Work out the finished part from the listing and answer in its coordinate system (mm). Coordinates: 2 decimals unless noted, no trailing zeros. Order: outer loops, then holes, each group sorted by start corner. A loop starts at its lowest first (then second) coordinate and runs counter-clockwise, first axis right, second up. Notation, with made-up numbers: (79.5, 11.25) - (136.5, 11.25) arc R23 cw to (136.5, 24.25) - close; hole circle Ø10 at (25, 55). An arc over 180 degrees is marked (long way). Answer as a JSON object with one key per item and string values. Group by question number.
1) Section D-D (x = 7) is taken. Give the vertices of the cut face in (y, z), plus the area to 3 significant figures.
2) Each of these flat-tipped pins is pushed along its axis until it touches: P1, Ø3, axis at x = -7.5, z = 19, coming from the -Y side; P2, Ø5, axis at x = 2.5, y = 2.5, coming from the +Z side; P3, Ø1.5, axis at y = 2, z = 13, coming from the -X side. Where does it stop, or does it pass through?
3) Section B-B (x = 16) is taken. Give the vertices of the cut face in (y, z).
4) Find the intervals of material crossed by line 1 along Y through (x, z) = (-13, 8.75); line 2 along Z through (x, y) = (-17, -2); line 3 along Z through (x, y) = (24, -4), in increasing order.
5) Section A-A (y = 3.75) is taken. Count the separate pieces of the cut face and the enclosed holes in it, plus the area to 3 significant figures.
from build123d import *

# Parameters (mm, degrees)
F1_DEPTH = 6.35
F2_DEPTH = 1.143
F0_R     = 0.5376774343
F3_DEPTH = 2.54


# Not quite as in the source:
# - a feature names something its author has since deleted; it is built from what else it names


with BuildPart() as f1:
    # F0 (on Front) → F1 (new body, symmetric)
    with BuildSketch(Plane.XZ):
        with BuildLine():
            Line((-23.957899441, 10.4580381471), (-18.3417778462, 24.3978608632))
            ThreePointArc((-18.3417778462, 24.3978608632), (-24.508682548, 21.9832418882), (-30.3090570475, 18.7868761299))
            ThreePointArc((-30.3090570475, 18.7868761299), (-30.4688345425, 18.7669734191), (-30.6283324456, 18.7449419699))
            ThreePointArc((-30.6283324456, 18.7449419699), (-33.5331514259, 15.8401229896), (-30.6283324456, 12.9353040093))
            ThreePointArc((-30.6283324456, 12.9353040093), (-29.7623700905, 12.8471763438), (-28.8964077355, 12.9353040093))
            ThreePointArc((-28.8964077355, 12.9353040093), (-26.4593844973, 11.6324177359), (-23.957899441, 10.4580381471))
        make_face()
    extrude(amount=F1_DEPTH, both=True)



with BuildPart() as f1b:
    # F0 (on Front) → F1, piece 2 (new body, symmetric)
    with BuildSketch(Plane.XZ):
        with BuildLine():
            Line((-18.3417778462, 8.3667041198), (-12.1646409942, 25.9439263056))
            ThreePointArc((-12.1646409942, 25.9439263056), (-14.2076271577, 25.5232665303), (-16.2316225469, 25.0190941641))
            Line((-16.2316225469, 25.0190941641), (-22.1410569955, 9.7018790977))
            Line((-22.1410569955, 9.7018790977), (-18.3417778462, 8.3667041198))
        make_face()
    extrude(amount=F1_DEPTH, both=True)


with BuildPart() as f1c:
    # F0 (on Front) → F1, piece 3 (new body, symmetric)
    with BuildSketch(Plane.XZ):
        with BuildLine():
            Line((1.8068482134, 6.1805279437), (6.278092768, 25.9439263056))
            ThreePointArc((6.278092768, 25.9439263056), (4.5833562732, 26.2272072808), (2.8800089407, 26.4530119809))
            Line((2.8800089407, 26.4530119809), (-1.8782013648, 5.999318733))
            Line((-1.8782013648, 5.999318733), (1.8068482134, 6.1805279437))
        make_face()
        with BuildLine():
            Line((-1.8782013648, 5.999318733), (2.8800089407, 26.4530119809))
            Line((2.8800089407, 26.4530119809), (0.4476490102, 26.6745825214))
            Line((0.4476490102, 26.6745825214), (-5.0909425313, 6.0502526163))
            ThreePointArc((-5.0909425313, 6.0502526163), (-3.4849571687, 6.0004872294), (-1.8782013648, 5.999318733))
        make_face()
    extrude(amount=F1_DEPTH, both=True)


with BuildPart() as f1d:
    # F0 (on Front) → F1, piece 4 (new body, symmetric)
    with BuildSketch(Plane.XZ):
        with BuildLine():
            Line((8.4127366642, 7.1570997269), (11.4288211982, 24.7124430234))
            ThreePointArc((11.4288211982, 24.7124430234), (9.992896211, 25.1131857412), (8.5458304529, 25.4716212117))
            Line((8.5458304529, 25.4716212117), (5.5570962218, 6.6305751818))
            Line((5.5570962218, 6.6305751818), (8.4127366642, 7.1570997269))
        make_face()
    extrude(amount=F1_DEPTH, both=True)


with BuildPart() as f1e:
    # F0 (on Front) → F1, piece 5 (new body, symmetric)
    with BuildSketch(Plane.XZ):
        with BuildLine():
            Line((15.3388230563, 9.1300772804), (17.0374851182, 22.6934409017))
            ThreePointArc((17.0374851182, 22.6934409017), (15.6698818595, 23.2551052755), (14.2865132328, 23.7767342476))
            Line((14.2865132328, 23.7767342476), (12.4090739429, 8.1711044117))
            Line((12.4090739429, 8.1711044117), (15.3388230563, 9.1300772804))
        make_face()
    extrude(amount=F1_DEPTH, both=True)


with BuildPart() as f1f:
    # F0 (on Front) → F1, piece 6 (new body, symmetric)
    with BuildSketch(Plane.XZ):
        with BuildLine():
            Line((21.0198694331, 18.0883333087), (21.0198694322, 20.7808247964))
            ThreePointArc((21.0198694322, 20.7808247964), (20.069859076, 21.2762433466), (19.1096116707, 21.7515160445))
            Line((19.1096116707, 21.7515160445), (17.6402366731, 10.0189484933))
            ThreePointArc((17.6402366731, 10.0189484933), (19.3434832269, 10.757776133), (21.0198694351, 11.5556761172))
            Line((21.0198694351, 11.5556761172), (21.0198694343, 14.3284648657))
            Line((21.0198694343, 14.3284648657), (21.0198694331, 18.0883333087))
        make_face()
        Polygon((21.0198694343, 14.3284648657), (28.0039037731, 15.6337103452), (21.0198694331, 18.0883333087), align=None)
    extrude(amount=F1_DEPTH, both=True)


with BuildPart() as f1_1:
    add(f1.part)

    add(f1b.part)  # F2 merges F1b

    add(f1c.part)  # F2 merges F1c

    add(f1d.part)  # F2 merges F1d

    add(f1e.part)  # F2 merges F1e

    add(f1f.part)  # F2 merges F1f
    # F0 (on Front) → F2 (join, symmetric)
    with BuildSketch(Plane.XZ):
        with BuildLine():
            Line((-12.1127719974, 6.8447730539), (-5.6567463208, 26.7153601349))
            ThreePointArc((-5.6567463208, 26.7153601349), (-6.3478066879, 26.6736702184), (-7.0382347309, 26.6225664263))
            Line((-7.0382347309, 26.6225664263), (-8.9119801903, 26.3745176413))
            Line((-8.9119801903, 26.3745176413), (-16.2316225469, 7.7613705689))
            ThreePointArc((-16.2316225469, 7.7613705689), (-14.1813025903, 7.2621558762), (-12.1127719974, 6.8447730539))
        make_face()
        with BuildLine():
            Line((-5.0909425313, 6.0502526163), (0.4476490102, 26.6745825214))
            ThreePointArc((0.4476490102, 26.6745825214), (-1.1501754418, 26.7562261377), (-2.7497784488, 26.787513187))
            Line((-2.7497784488, 26.787513187), (-9.4000246121, 6.4253498282))
            ThreePointArc((-9.4000246121, 6.4253498282), (-9.0947770245, 6.3870993561), (-8.7893130258, 6.3506173901))
            ThreePointArc((-8.7893130258, 6.3506173901), (-7.91449717, 6.2560428931), (-7.0382347309, 6.1759725811))
            ThreePointArc((-7.0382347309, 6.1759725811), (-6.0651659933, 6.1041697642), (-5.0909425313, 6.0502526163))
        make_face()
        with BuildLine():
            Line((-9.4000246121, 6.4253498282), (-2.7497784488, 26.787513187))
            ThreePointArc((-2.7497784488, 26.787513187), (-2.8593531847, 26.7878123797), (-2.968928311, 26.7878752202))
            Line((-2.968928311, 26.7878752202), (-5.6567463208, 26.7153601349))
            Line((-5.6567463208, 26.7153601349), (-12.1127719974, 6.8447730539))
            ThreePointArc((-12.1127719974, 6.8447730539), (-10.7591081046, 6.6175349855), (-9.4000246121, 6.4253498282))
        make_face()
        with BuildLine():
            ThreePointArc((-18.3417778462, 8.3667041198), (-17.2898277228, 8.0531349816), (-16.2316225469, 7.7613705689))
            Line((-16.2316225469, 7.7613705689), (-8.9119801903, 26.3745176413))
            Line((-8.9119801903, 26.3745176413), (-12.1646409942, 25.9439263056))
            Line((-12.1646409942, 25.9439263056), (-18.3417778462, 8.3667041198))
        make_face()
        with BuildLine():
            Line((5.5570962218, 6.6305751818), (8.5458304529, 25.4716212117))
            Line((8.5458304529, 25.4716212117), (6.278092768, 25.9439263056))
            Line((6.278092768, 25.9439263056), (1.8068482134, 6.1805279437))
            ThreePointArc((1.8068482134, 6.1805279437), (3.6859738146, 6.3722062161), (5.5570962218, 6.6305751818))
        make_face()
        with BuildLine():
            Line((12.4090739429, 8.1711044117), (14.2865132328, 23.7767342476))
            Line((14.2865132328, 23.7767342476), (11.4288211982, 24.7124430234))
            Line((11.4288211982, 24.7124430234), (8.4127366642, 7.1570997269))
            ThreePointArc((8.4127366642, 7.1570997269), (10.4207473928, 7.62531299), (12.4090739429, 8.1711044117))
        make_face()
        with BuildLine():
            Line((17.6402366731, 10.0189484933), (19.1096116707, 21.7515160445))
            Line((19.1096116707, 21.7515160445), (17.0374851182, 22.6934409017))
            Line((17.0374851182, 22.6934409017), (15.3388230563, 9.1300772804))
            ThreePointArc((15.3388230563, 9.1300772804), (16.4946911486, 9.5611495909), (17.6402366731, 10.0189484933))
        make_face()
        with BuildLine():
            Line((-22.1410569955, 9.7018790977), (-16.2316225469, 25.0190941641))
            ThreePointArc((-16.2316225469, 25.0190941641), (-17.2900631098, 24.7199003867), (-18.3417778462, 24.3978608632))
            Line((-18.3417778462, 24.3978608632), (-23.957899441, 10.4580381471))
            ThreePointArc((-23.957899441, 10.4580381471), (-23.0529803303, 10.0715440095), (-22.1410569955, 9.7018790977))
        make_face()
    extrude(amount=F2_DEPTH, both=True)

    # F0 (on Front) → F3 (join, symmetric)
    with BuildSketch(Plane.XZ):
        with BuildLine():
            Line((-22.1410569955, 9.7018790977), (-16.2316225469, 25.0190941641))
            ThreePointArc((-16.2316225469, 25.0190941641), (-17.2900631098, 24.7199003867), (-18.3417778462, 24.3978608632))
            Line((-18.3417778462, 24.3978608632), (-23.957899441, 10.4580381471))
            ThreePointArc((-23.957899441, 10.4580381471), (-23.0529803303, 10.0715440095), (-22.1410569955, 9.7018790977))
        make_face()
        with BuildLine():
            ThreePointArc((-18.3417778462, 8.3667041198), (-17.2898277228, 8.0531349816), (-16.2316225469, 7.7613705689))
            Line((-16.2316225469, 7.7613705689), (-8.9119801903, 26.3745176413))
            Line((-8.9119801903, 26.3745176413), (-12.1646409942, 25.9439263056))
            Line((-12.1646409942, 25.9439263056), (-18.3417778462, 8.3667041198))
        make_face()
        with BuildLine():
            Line((-9.4000246121, 6.4253498282), (-2.7497784488, 26.787513187))
            ThreePointArc((-2.7497784488, 26.787513187), (-2.8593531847, 26.7878123797), (-2.968928311, 26.7878752202))
            Line((-2.968928311, 26.7878752202), (-5.6567463208, 26.7153601349))
            Line((-5.6567463208, 26.7153601349), (-12.1127719974, 6.8447730539))
            ThreePointArc((-12.1127719974, 6.8447730539), (-10.7591081046, 6.6175349855), (-9.4000246121, 6.4253498282))
        make_face()
        with BuildLine():
            Line((5.5570962218, 6.6305751818), (8.5458304529, 25.4716212117))
            Line((8.5458304529, 25.4716212117), (6.278092768, 25.9439263056))
            Line((6.278092768, 25.9439263056), (1.8068482134, 6.1805279437))
            ThreePointArc((1.8068482134, 6.1805279437), (3.6859738146, 6.3722062161), (5.5570962218, 6.6305751818))
        make_face()
        with BuildLine():
            Line((12.4090739429, 8.1711044117), (14.2865132328, 23.7767342476))
            Line((14.2865132328, 23.7767342476), (11.4288211982, 24.7124430234))
            Line((11.4288211982, 24.7124430234), (8.4127366642, 7.1570997269))
            ThreePointArc((8.4127366642, 7.1570997269), (10.4207473928, 7.62531299), (12.4090739429, 8.1711044117))
        make_face()
        with BuildLine():
            Line((17.6402366731, 10.0189484933), (19.1096116707, 21.7515160445))
            Line((19.1096116707, 21.7515160445), (17.0374851182, 22.6934409017))
            Line((17.0374851182, 22.6934409017), (15.3388230563, 9.1300772804))
            ThreePointArc((15.3388230563, 9.1300772804), (16.4946911486, 9.5611495909), (17.6402366731, 10.0189484933))
        make_face()
        Polygon((28.0039037731, 15.6337103452), (21.0198694322, 20.7808247964), (21.0198694331, 18.0883333087), align=None)
        Polygon((21.0198694351, 11.5556761172), (28.0039037731, 15.6337103452), (21.0198694343, 14.3284648657), align=None)
        with BuildLine():
            ThreePointArc((-18.3417778462, 24.3978608632), (-17.2900631098, 24.7199003867), (-16.2316225469, 25.0190941641))
            Line((-16.2316225469, 25.0190941641), (-16.2316225469, 27.5203254709))
            Line((-16.2316225469, 27.5203254709), (-18.3417778462, 27.6264417917))
            Line((-18.3417778462, 27.6264417917), (-18.3417778462, 24.3978608632))
        make_face()
        with BuildLine():
            Line((-18.3417778462, 27.6264417917), (-16.2316225469, 27.5203254709))
            ThreePointArc((-16.2316225469, 27.5203254709), (-17.1834027814, 29.6274841361), (-18.3417778462, 27.6264417917))
        make_face()
        with Locations((-17.248678008, 28.3294664105)):
            Circle(F0_R, mode=Mode.SUBTRACT)
        with BuildLine():
            Line((-6.263176576, 3.5358044787), (-7.0382347309, 6.1759725811))
            ThreePointArc((-7.0382347309, 6.1759725811), (-7.91449717, 6.2560428931), (-8.7893130258, 6.3506173901))
            Line((-8.7893130258, 6.3506173901), (-7.8281190425, 3.0763937997))
            Line((-7.8281190425, 3.0763937997), (-6.263176576, 3.5358044787))
        make_face()
        with BuildLine():
            Line((-6.4755459316, 3.2506433781), (-6.263176576, 3.5358044787))
            Line((-6.263176576, 3.5358044787), (-7.8281190425, 3.0763937997))
            ThreePointArc((-7.8281190425, 3.0763937997), (-7.1834055221, 1.5302282542), (-5.857669426, 2.5542923249))
            Line((-5.857669426, 2.5542923249), (-6.0594304827, 3.2415737925))
            Line((-6.0594304827, 3.2415737925), (-6.6755125299, 2.7018676046))
            Line((-6.6755125299, 2.7018676046), (-6.8233669735, 2.54364172))
            Line((-6.8233669735, 2.54364172), (-6.2799803729, 2.3477658746))
            Line((-6.2799803729, 2.3477658746), (-6.9631087507, 2.1509963489))
            Line((-6.9631087507, 2.1509963489), (-7.4357455596, 2.5542923249))
            Line((-7.4357455596, 2.5542923249), (-7.3302290402, 2.8919170145))
            Line((-7.3302290402, 2.8919170145), (-6.4755459316, 3.2506433781))
        make_face()
    extrude(amount=F3_DEPTH, both=True)


solid = f1_1.part
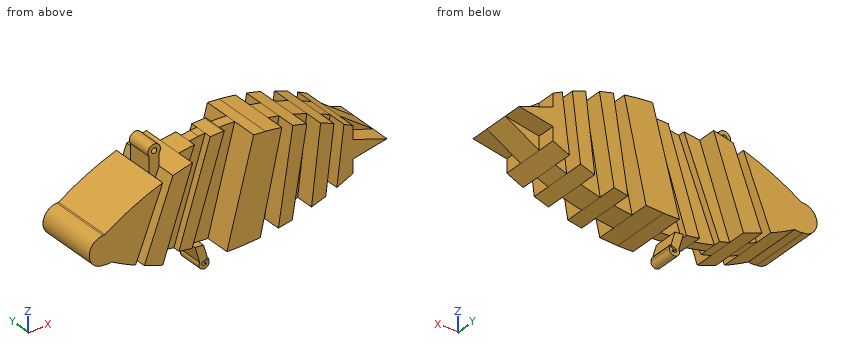
Report:
{
 "1": {"outline": "(-6.35, 6.9) - (6.35, 6.9) - (6.35, 15.73) - (2.54, 15.73) - (2.54, 25.79) - (-2.54, 25.79) - (-2.54, 15.73) - (-6.35, 15.73) - close", "area": "163 mm²"},
 "2": {"P1": "stops at y = -2.54", "P2": "stops at z = 26.68", "P3": "stops at x = -32.65"},
 "3": {"outline": "(-6.35, 14.41) - (-2.54, 14.41) - (-2.54, 9.37) - (2.54, 9.37) - (2.54, 14.41) - (6.35, 14.41) - (6.35, 23.12) - (-6.35, 23.12) - close"},
 "4": {"line 1": "y = -1.14 to 1.14", "line 2": "z = 7.97 to 27.85, 28.81 to 29.61", "line 3": "z = 14.89 to 17.04"},
 "5": {"separate pieces": "6", "enclosed holes": "0", "area": "436 mm²"}
}
